Part model, mm, in its own coordinate system. Coordinates: 2 decimals unless noted, no trailing zeros. Write each loop counter-clockwise with the first axis right and the second up, starting at its lowest first coordinate (ties: lowest second). Pieces come first, ordered by that corner, then holes. Notation, with made-up numbers: (62, 26.25) -> (68, 26.25) arc R10 cw to (68, 35.25) -> close; hole circle Ø2 at (68, 39). An arc over 180 degrees is marked (long way). Write item = value, one per line. Start each with the question number.
Q1. Band-saw the part on D-D, the plane x = 0. List the corners of the cut face in (y, z), plus the area to 3 significant figures.
Q2. Probe line 1 (Y direction, x = -16.5, z = 3); line 2 (X direction, y = -16.5, z = 5.25); line 3 (X direction, y = 0.5, z = 8). List the from-to ranges inside material, lowest first.
Q3. Pin check, flat tip, straight feed: P1, Ø6.5, axis at x = -16.5, y = 29, coming from the -Z side. Stop position of the tip, or through.
Q4. Band-saw the part on B-B, the plane y = -29. List the corners of the cut face in (x, z).
Q5. Pull direction X, two halves, no side cores. Call faces 1 (the cylindrical face through (-16.04, -32.47, 4.93)), 2 (the flat face through (-11, 9, 10)), 3 (the cylindrical face through (-24.287, 39.248, 5.07)): released by +X, released by -X, zero draft, split by the parting line, or undercut.
Q6. Band-saw the part on C-C, the plane z = 8.5. Give the number of separate pieces and of enclosed holes in the cut face, plus the area to 3 significant figures.
Q7. Band-saw the part on A-A, the plane x = -16.5. List the corners of the cut face in (y, z).
from build123d import *

# Parameters (mm, degrees)
SKETCH_2_W                 = 50
SKETCH_2_H                 = 80
EXTRUDE_1_DEPTH            = 10
SKETCH_3_R                 = 3.5
SKETCH_3_R_2               = 3
CUT_EXTRUDE_1_DEPTH        = 49.218253805
MIRROR_2_COPY_1_SKETCH_R   = 3.5
MIRROR_2_COPY_1_SKETCH_R_2 = 3
MIRROR_2_COPY_1_DEPTH      = 49.218253805
SKETCH_4_R                 = 14
CUT_EXTRUDE_2_DEPTH        = 49.218253805
FILLET_1_R                 = 2.5


with BuildPart() as part:
    # 草图2 → 凸台-拉伸1 (new body)
    with BuildSketch(Plane.XY):
        Rectangle(SKETCH_2_W, SKETCH_2_H)
    extrude(amount=EXTRUDE_1_DEPTH)

    # 草图3 → 切除-拉伸1 (cut, through all)
    with BuildSketch(Plane(origin=(0, 0, 0), x_dir=(-1, 0, 0), z_dir=(0, 0, -1))):
        with Locations((16.5, 29)):
            Circle(SKETCH_3_R)
        with Locations((16.5, 16.5)):
            Circle(SKETCH_3_R_2)
    cut_extrude_1 = extrude(amount=-CUT_EXTRUDE_1_DEPTH, mode=Mode.SUBTRACT)

    # 镜向1: 切除-拉伸1 across plane
    add(cut_extrude_1.mirror(Plane(origin=(0, 0, 0), x_dir=(0, 0, 1), z_dir=(1, 0, 0))), mode=Mode.SUBTRACT)

    # 镜向2: 切除-拉伸1 across plane
    add(cut_extrude_1.mirror(Plane.ZX), mode=Mode.SUBTRACT)

    # 镜向2 copy 1 sketch → 镜向2 copy 1 (cut, through all)
    with BuildSketch(Plane(origin=(0, 0, 0), x_dir=(1, 0, 0), z_dir=(0, 0, -1))):
        with Locations((16.5, 29)):
            Circle(MIRROR_2_COPY_1_SKETCH_R)
        with Locations((16.5, 16.5)):
            Circle(MIRROR_2_COPY_1_SKETCH_R_2)
    extrude(amount=-MIRROR_2_COPY_1_DEPTH, mode=Mode.SUBTRACT)

    # 草图4 → 切除-拉伸2 (cut, through all)
    with BuildSketch(Plane(origin=(0, 0, 0), x_dir=(-1, 0, 0), z_dir=(0, 0, -1))):
        Circle(SKETCH_4_R)
    extrude(amount=-CUT_EXTRUDE_2_DEPTH, mode=Mode.SUBTRACT)

    # 圆角1
    fillet_1_edges = [part.edges().sort_by_distance(p)[0] for p in [
        (-25, 40, 5),
        (25, 40, 5),
        (25, -40, 5),
        (-25, -40, 5),
    ]]
    fillet(fillet_1_edges, radius=FILLET_1_R)


solid = part.part
Ans:
q1.outline = (-40, 0) -> (-14, 0) -> (-14, 10) -> (-40, 10) -> close; (14, 0) -> (40, 0) -> (40, 10) -> (14, 10) -> close
q1.area = 520 mm2
q2.line_1 = -40 to -32.5, -25.5 to -19.5, -13.5 to 13.5, 19.5 to 25.5, 32.5 to 40
q2.line_2 = -25 to -19.5, -13.5 to 13.5, 19.5 to 25
q2.line_3 = -25 to -13.99, 13.99 to 25
q3.P1 = through
q4.outline = (-25, 0) -> (-20, 0) -> (-20, 10) -> (-25, 10) -> close; (-13, 0) -> (13, 0) -> (13, 10) -> (-13, 10) -> close; (20, 0) -> (25, 0) -> (25, 10) -> (20, 10) -> close
q5.face_1 = undercut
q5.face_2 = zero draft
q5.face_3 = released by -X
q6.separate_pieces = 1
q6.enclosed_holes = 9
q6.area = 3,110 mm2
q7.outline = (-40, 0) -> (-32.5, 0) -> (-32.5, 10) -> (-40, 10) -> close; (-25.5, 0) -> (-19.5, 0) -> (-19.5, 10) -> (-25.5, 10) -> close; (-13.5, 0) -> (13.5, 0) -> (13.5, 10) -> (-13.5, 10) -> close; (19.5, 0) -> (25.5, 0) -> (25.5, 10) -> (19.5, 10) -> close; (32.5, 0) -> (40, 0) -> (40, 10) -> (32.5, 10) -> close
